Can you work these out from the model? Positions are in its coordinate system, mm. A direction names the side the tool comes from. Give positions to 0.01 mm unless a question says otherwise; leave off trailing zeros. Loops run counter-clockwise (first coordinate to the right, second up) from the corner with the lowest first, then second, coordinate; pieces in that order, holes last. Notation, with made-up numbers: M 49.25,-6 L 90.25,-6 A18 ccw 90.25,25 Z; hole C -39.75,40.5 d8. An arc over 180 degrees is marked long. One line per item, written item: value. Start each with the question number.
from build123d import *

# Parameters (mm, degrees)
F0_R     = 19.05
F1_DEPTH = 457.2
F2_SIZE2 = 1.5875
F2_SIZE  = 1.5875
F4_DEPTH = 19.05


# Not quite as in the source:
# - a pattern or mirror of a feature is missing from the dataset's text; its kind, count and spacing are read off the source's solid


with BuildPart() as f1:
    # F0 (on Top) → F1 (new body, symmetric)
    with BuildSketch(Plane.XY):
        Circle(F0_R)
    extrude(amount=F1_DEPTH, both=True)

    # F2
    f2_edges = [f1.edges().sort_by_distance(p)[0] for p in [
        (-19.05, 0, 457.2),
        (-19.05, 0, -457.2),
    ]]
    chamfer(f2_edges, length=F2_SIZE, length2=F2_SIZE2)

    # F3 (on Front) → F4 (cut, symmetric)
    with BuildSketch(Plane.XZ):
        with BuildLine():
            Line((4.7752, 292.1), (4.7752, -292.1))
            ThreePointArc((4.7752, -292.1), (17.4752, -304.8), (30.1752, -292.1))
            Line((30.1752, -292.1), (30.1752, 292.1))
            ThreePointArc((30.1752, 292.1), (17.4752, 304.8), (4.7752, 292.1))
        make_face()
    f4 = extrude(amount=F4_DEPTH, both=True, mode=Mode.SUBTRACT)

    # F4_copies: F4 across plane
    add(f4.mirror(Plane(origin=(0, 0, 0), x_dir=(0, 0, -1), z_dir=(-1, 0, 0))), mode=Mode.SUBTRACT)


solid = f1.part
Q1. I need wall thicknesses on line 1 along Z through (x, y) = (15.5, -8); line 2 along X through (y, z) = (-4, -19.5); line 3 along Z through (x, y) = (-11, -7). Which ranges of each line are inside material? Lowest first, please.
Q2. Which directions (+Z, -Z, +X, -X, +Y, -Y) give clear straight access to the entire face, cutting with the end or side of a thin tool? Please do faces 4 (the face through (4.775, 0, 4)), 5 (the face through (-4.775, 0, 4)), 6 (the face through (-2.48, 18.888, 107.626)).
Q3. If we section it at A-A, the plane y = 0: Write out the boundary of the cut face in (x, z).
Q4. If we section it at B-B, the plane z = 6.5: Write out the boundary of the cut face in (x, y), plus the area to 3 significant figures.
Q5. If we mould it in two halves opening along Z, with no side actions, what happens to faces 1 (the face through (0, 0, 457.2)), 2 (the face through (0, 0, -457.2)), 3 (the face through (-7.53, -0.26, 300))? For each: released by +Z, released by -Z, zero draft, split by the parting line, or undercut.
Q6. For P1, Ø12, axis at x = -4, z = 211, coming from the -Y side; P2, Ø8, axis at y = 10, z = -131.5, coming from the -X side; P3, Ø8, axis at y = -11, z = 303, coming from the +X side, each with a flat end and sliding along its axis, tell me the tip position at first contact or that it passes through.
Q7. If we section it at C-C, the plane z = -391: Write out the boundary of the cut face in (x, y).
Response:
1. line 1: -457.2 to -304.65, 304.65 to 457.2
1. line 2: -4.78 to 4.78
1. line 3: -457.2 to -303.03, 303.03 to 457.2
2. face 4: +X, +Y, -Y
2. face 5: -X, +Y, -Y
2. face 6: +Z, -Z
3. outline: M -19.05,-455.61 L -17.46,-457.2 L 17.46,-457.2 L 19.05,-455.61 L 19.05,-304.7 A12.7 cw 4.78,-292.1 L 4.78,292.1 A12.7 cw 19.05,304.7 L 19.05,455.61 L 17.46,457.2 L -17.46,457.2 L -19.05,455.61 L -19.05,304.7 A12.7 cw -4.78,292.1 L -4.78,-292.1 A12.7 cw -19.05,-304.7 Z
4. outline: M -4.78,-18.44 A19.05 ccw 4.78,-18.44 L 4.78,18.44 A19.05 ccw -4.78,18.44 Z
4. area: 360 mm^2
5. face 1: released by +Z
5. face 2: released by -Z
5. face 3: undercut
6. P1: y = -19.05
6. P2: x = -4.78
6. P3: x = 17.54
7. outline: C 0,0 d38.1
